```python
from build123d import *

# Parameters (mm, degrees)
F0_W     = 668
F0_H     = 60
F0_R     = 10
F1_DEPTH = 25
F2_R     = 20
F3_R     = 20
F4_R     = 20
F5_R     = 20


with BuildPart() as f1:
    # F0 (on Right) → F1 (new body)
    with BuildSketch(Plane.YZ):
        with Locations((247.531975, 0)):
            Rectangle(F0_W, F0_H)
        with Locations((-56.468025, 0)):
            Circle(F0_R, mode=Mode.SUBTRACT)
        with Locations((551.531975, 0)):
            Circle(F0_R, mode=Mode.SUBTRACT)
    extrude(amount=F1_DEPTH)

    # F2
    f2_edges = [f1.edges().sort_by_distance(p)[0] for p in [
        (12.5, 581.531975, 30),
    ]]
    fillet(f2_edges, radius=F2_R)

    # F3
    f3_edges = [f1.edges().sort_by_distance(p)[0] for p in [
        (12.5, 581.531975, -30),
    ]]
    fillet(f3_edges, radius=F3_R)

    # F4
    f4_edges = [f1.edges().sort_by_distance(p)[0] for p in [
        (12.5, -86.468025, 30),
    ]]
    fillet(f4_edges, radius=F4_R)

    # F5
    f5_edges = [f1.edges().sort_by_distance(p)[0] for p in [
        (12.5, -86.468025, -30),
    ]]
    fillet(f5_edges, radius=F5_R)


solid = f1.part
```
Model file for the job. Use its own axes, mm. Coordinates: 2 decimals unless noted, no trailing zeros. Loops run counter-clockwise (first coordinate to the right, second up) from the corner with the lowest first, then second, coordinate; pieces in that order, holes last. Notation, with made-up numbers: (79.25, 6) - (107.25, 6) arc R14 ccw to (107.25, 15) - close; hole circle Ø2 at (42, 20). An arc over 180 degrees is marked (long way). Answer as a JSON object with one key per item and string values. Group by question number.
(1) Flat gauge pins, fed straight in: pin 1 (5 mm diameter, centred on y = 399, z = 19, fed in from -X); pin 2 (10 mm diameter, centred on x = 14.5, z = 20, fed in from +Y). Where does each tip first touch, or does it go through?
(2) Cut at B-B (x = 5). Give the cut face in (y, z), then the cut area to 3 significant figures.
(3) Probe line 1 along Z through (x, y) = (6.75, 547); line 2 along Y through (x, z) = (7, -13); line 3 along Y through (x, z) = (8.75, 19). List the from-to ranges inside material, lowest first.
(4) Cut at C-C (z = -24). Give the cut face in (x, y), then the cut area to 3 significant figures.
(5) Cut at A-A (z = 0). Give the cut face in (x, y).
(6) Two-plate mould, pull along Y, no slides. Class faces 1 (the face through (12.68, -80.45, 24.3)), 2 (the face through (25, 243, 0)), 3 (the face through (12.675, 575.829, -23.986)), 4 (the face through (12.32, 541.54, 0.44)): released by +Y, released by -Y, zero draft, split by the parting line, or undercut.
Geometry says:
{
 "1": {"pin 1": "stops at x = 0", "pin 2": "stops at y = 580.9"},
 "2": {"outline": "(-86.47, -10) arc R20 ccw to (-66.47, -30) - (561.53, -30) arc R20 ccw to (581.53, -10) - (581.53, 10) arc R20 ccw to (561.53, 30) - (-66.47, 30) arc R20 ccw to (-86.47, 10) - close; hole circle Ø20 at (-56.47, 0); hole circle Ø20 at (551.53, 0)", "area": "39,100 mm^2"},
 "3": {"line 1": "z = -30 to -8.91, 8.91 to 30", "line 2": "y = -86.24 to 581.31", "line 3": "y = -84.33 to 579.39"},
 "4": {"outline": "(0, -80.75) - (25, -80.75) - (25, 575.81) - (0, 575.81) - close", "area": "16,400 mm^2"},
 "5": {"outline": "(0, -86.47) - (25, -86.47) - (25, -66.47) - (0, -66.47) - close; (0, -46.47) - (25, -46.47) - (25, 541.53) - (0, 541.53) - close; (0, 561.53) - (25, 561.53) - (25, 581.53) - (0, 581.53) - close"},
 "6": {"face 1": "released by -Y", "face 2": "zero draft", "face 3": "released by +Y", "face 4": "undercut"}
}
